Build history of the part. All positions in model axes, mm. A direction names the side the tool comes from. Give positions to 0.01 mm unless a question says otherwise; leave off trailing zeros. Write each loop counter-clockwise with the first axis right and the second up, starting at its lowest first coordinate (ties: lowest second). Pieces come first, ordered by that corner, then holes. Notation, with made-up numbers: (86, 22) -> (103, 22) arc R20 ccw to (103, 32) -> close; hole circle Ø8 at (-9, -38.5). An arc over 180 degrees is marked (long way). Put each result on its own line as item: value.
from build123d import *

# Parameters (mm, degrees)
F0_W      = 32
F0_H      = 32
F1_DEPTH  = 20
F2_R      = 4
F3_DEPTH  = 4
F4_R      = 4
F5_DEPTH  = 4
F7_R      = 4
F8_DEPTH  = 4
F10_R     = 4
F11_DEPTH = 4
F12_R     = 0.2
F13_R     = 0.2
F14_R     = 0.2
F15_R     = 0.2


with BuildPart() as f1:
    # F0 (on Top) → F1 (new body)
    with BuildSketch(Plane.XY):
        with Locations((20.307853, -9.500817)):
            Rectangle(F0_W, F0_H)
    extrude(amount=F1_DEPTH)

    # F2 (on face) → F3 (join)
    with BuildSketch(Plane.XY.offset(20)):
        with Locations((12.307853, 0)):
            Circle(F2_R)
    extrude(amount=F3_DEPTH)

    # F4 (on face) → F5 (join)
    with BuildSketch(Plane.XY.offset(20)):
        with Locations((28.307853, 0)):
            Circle(F4_R)
    extrude(amount=F5_DEPTH)

    # F7 (on face) → F8 (join)
    with BuildSketch(Plane.XY.offset(20)):
        with Locations((12.307853, -17.500817)):
            Circle(F7_R)
    extrude(amount=F8_DEPTH)

    # F10 (on face) → F11 (join)
    with BuildSketch(Plane.XY.offset(20)):
        with Locations((28.307853, -17.500817)):
            Circle(F10_R)
    extrude(amount=F11_DEPTH)

    # F12
    f12_edges = [f1.edges().sort_by_distance(p)[0] for p in [
        (8.307853, 0, 24),
    ]]
    fillet(f12_edges, radius=F12_R)

    # F13
    f13_edges = [f1.edges().sort_by_distance(p)[0] for p in [
        (8.307853, -17.500817, 24),
    ]]
    fillet(f13_edges, radius=F13_R)

    # F14
    f14_edges = [f1.edges().sort_by_distance(p)[0] for p in [
        (24.307853, -17.500817, 24),
    ]]
    fillet(f14_edges, radius=F14_R)

    # F15
    f15_edges = [f1.edges().sort_by_distance(p)[0] for p in [
        (24.307853, 0, 24),
    ]]
    fillet(f15_edges, radius=F15_R)


solid = f1.part
1) Tool access for faces 4 (the flat face through (20, -9, 20)), 5 (the flat face through (20, -9, 0)): list every direction of +Z, -Z, +X, -X, +Y, -Y with a clear straight run to the whole face (end or side of a thin tool).
Filled sheet:
face 4: +Z
face 5: -Z, +X, -X, +Y, -Y
2) Pull direction Y, two halves, no side cores. Call faces 1 (the flat face through (20, -25.501, 10)), 2 (the cylindrical face through (9.13, -2.43, 21.87)), 3 (the flat face through (28, -17, 24)): released by +Y, released by -Y, zero draft, split by the parting line, or undercut.
Filled sheet:
face 1: released by -Y
face 2: undercut
face 3: zero draft
3) Slice it at B-B (x = 22). Write the cut outline in (y, z).
Filled sheet:
outline: (-25.5, 0) -> (6.5, 0) -> (6.5, 20) -> (-25.5, 20) -> close
4) Wall check: L1, parallel to Y at x = 12.5, z = 22.75; L2, parallel to Z at x = 16.5, y = -7.5; L3, parallel to Z at x = 32, y = -16.5. Give the ranges that are in metal, low to high.
Filled sheet:
L1: -21.5 to -13.51, -4 to 4
L2: 0 to 20
L3: 0 to 24
5) Slice it at A-A (y = 0). Write the cut outline in (x, z).
Filled sheet:
outline: (4.31, 0) -> (36.31, 0) -> (36.31, 20) -> (32.31, 20) -> (32.31, 23.8) arc R0.2 ccw to (32.11, 24) -> (24.51, 24) arc R0.2 ccw to (24.31, 23.8) -> (24.31, 20) -> (16.31, 20) -> (16.31, 23.8) arc R0.2 ccw to (16.11, 24) -> (8.51, 24) arc R0.2 ccw to (8.31, 23.8) -> (8.31, 20) -> (4.31, 20) -> close
6) Slice it at C-C (y = -4.5). Write the cut outline in (x, z), plus the area to 3 significant figures.
Filled sheet:
outline: (4.31, 0) -> (36.31, 0) -> (36.31, 20) -> (4.31, 20) -> close
area: 640 mm2
